from build123d import *

# Parameters (mm, degrees)
SKETCH_1_R      = 1.5
EXTRUDE_1_DEPTH = 5


with BuildPart() as part:
    # 스케치1 → 보스-돌출1 (new body)
    # profile 1 of 5: a face of its own
    with BuildSketch(Plane.XY):
        with BuildLine():
            Line((27.83772234, 1.5), (3.16227766, 1.5))
            ThreePointArc((3.16227766, 1.5), (3.414525722, 0.768774411), (3.5, 0))
            ThreePointArc((3.5, 0), (3.414525722, -0.768774411), (3.16227766, -1.5))
            Line((3.16227766, -1.5), (27.83772234, -1.5))
            ThreePointArc((27.83772234, -1.5), (27.5, 0), (27.83772234, 1.5))
        make_face()
    # profile 2 of 5: a face of its own
    with BuildSketch(Plane.XY):
        with BuildLine():
            ThreePointArc((3.16227766, 1.5), (1.870828693, 2.958039892), (0, 3.5))
            ThreePointArc((0, 3.5), (-3.5, 0), (0, -3.5))
            ThreePointArc((0, -3.5), (1.870828693, -2.958039892), (3.16227766, -1.5))
            Line((3.16227766, -1.5), (3.16227766, 1.5))
        make_face()
        Circle(SKETCH_1_R, mode=Mode.SUBTRACT)
    # profile 3 of 5: a face of its own
    with BuildSketch(Plane.XY):
        with BuildLine():
            ThreePointArc((34.5, 0), (33.474873734, 2.474873734), (31, 3.5))
            ThreePointArc((31, 3.5), (29.129171307, 2.958039892), (27.83772234, 1.5))
            Line((27.83772234, 1.5), (27.83772234, -1.5))
            ThreePointArc((27.83772234, -1.5), (29.129171307, -2.958039892), (31, -3.5))
            ThreePointArc((31, -3.5), (33.474873734, -2.474873734), (34.5, 0))
        make_face()
        with Locations((31, 0)):
            Circle(SKETCH_1_R, mode=Mode.SUBTRACT)
    # profile 4 of 5: a face of its own
    with BuildSketch(Plane.XY):
        with BuildLine():
            ThreePointArc((3.5, 0), (3.414525722, 0.768774411), (3.16227766, 1.5))
            Line((3.16227766, 1.5), (3.16227766, -1.5))
            ThreePointArc((3.16227766, -1.5), (3.414525722, -0.768774411), (3.5, 0))
        make_face()
    # profile 5 of 5: a face of its own
    with BuildSketch(Plane.XY):
        with BuildLine():
            Line((27.83772234, -1.5), (27.83772234, 1.5))
            ThreePointArc((27.83772234, 1.5), (27.5, 0), (27.83772234, -1.5))
        make_face()
    extrude(amount=EXTRUDE_1_DEPTH)


solid = part.part
The listing builds one solid part. Answer for the finished solid, in the listing's coordinates (mm). A direction names the side the tool comes from. Round coordinates to 2 decimals unless told otherwise and drop trailing zeros. Loops run counter-clockwise (first coordinate to the right, second up) from the corner with the lowest first, then second, coordinate; pieces in that order, holes last. Notation, with made-up numbers: M 73,13.25 L 89,13.25 A19 ccw 89,31.25 Z; hole C 46.25,-19 d3. An arc over 180 degrees is marked long. Return JSON: item names as keys, results as strings.
Q1. Find the intervals of material crossed by line 1 along Y through (x, z) = (31, 2.1); line 2 along X through (y, z) = (1, 3.4); line 3 along X through (y, z) = (1.25, 3), in increasing order. Write a range as from..to.
Results list:
{"line 1": "y = -3.5..-1.5, 1.5..3.5", "line 2": "x = -3.35..-1.12, 1.12..29.88, 32.12..34.35", "line 3": "x = -3.27..-0.83, 0.83..30.17, 31.83..34.27"}
Q2. Which of the six approach directions +Z, -Z, +X, -X, +Y, -Y give full straight-line access (tool end or side, diameter ignored) to faces 1 (the face through (16, 1.5, 2)), 2 (the face through (29.5, 0.07, 2.46))?
Results list:
{"face 1": "+Z, -Z, +Y", "face 2": "+Z, -Z"}
Q3. The mould has two halves that part along Y. Classify faces 3 (the face through (15, 0, 5)), 4 (the face through (15, -1.5, 2)), 5 (the face through (-1.5, 0.07, 2.46)): released by +Y, released by -Y, zero draft, split by the parting line, or undercut.
Results list:
{"face 3": "zero draft", "face 4": "released by -Y", "face 5": "undercut"}
Q4. Find section C-C, the plane x = 13.5. Determine the outline of the cut face in (y, z), plus the area to 3 significant figures.
Results list:
{"outline": "M -1.5,0 L 1.5,0 L 1.5,5 L -1.5,5 Z", "area": "15.0 mm2"}
Q5. Each of these flat-tipped pins is pushed along its axis until it touches: pin 1 Ø1 at (x, z) = (15, 3) entering from +Y; pin 2 Ø4 at (x, y) = (0, 0) entering from +Z. Where does it stop, or does it pass through?
Results list:
{"pin 1": "stops at y = 1.5", "pin 2": "stops at z = 5"}
Q6. Find section B-B, the plane y = 2. Determine the outline of the cut face in (x, z).
Results list:
{"outline": "M -2.87,0 L 2.87,0 L 2.87,5 L -2.87,5 Z; M 28.13,0 L 33.87,0 L 33.87,5 L 28.13,5 Z"}
Q7. Find section A-A, the plane z = 2. Determine the outline of the cut face in (x, y).
Results list:
{"outline": "M 3.16,-1.5 L 27.84,-1.5 A3.5 ccw long 27.84,1.5 L 3.16,1.5 A3.5 ccw long Z; hole C 0,0 d3; hole C 31,0 d3"}
